from build123d import *

# Parameters (mm, degrees)
SKETCH1_W           = 14.15
SKETCH1_H           = 44.35
BOSS_EXTRUDE1_DEPTH = 1.19
SKETCH2_R           = 0.625
CUT_EXTRUDE1_DEPTH  = 24.306701826
SKETCH3_R           = 0.75
CUT_EXTRUDE2_DEPTH  = 24.306701826
SKETCH4_W           = 5
SKETCH4_H           = 4
BOSS_EXTRUDE2_DEPTH = 1.5
SKETCH4_3_W         = 1.75
SKETCH4_3_H         = 3.5
BOSS_EXTRUDE3_DEPTH = 1.65
SKETCH7_W           = 1.25
SKETCH7_H           = 2.5
BOSS_EXTRUDE6_DEPTH = 0.5


with BuildPart() as part:
    # Sketch1 → Boss-Extrude1 (new body)
    with BuildSketch(Plane(origin=(0, 0, 0), x_dir=(1, 0, 0), z_dir=(0, 1, 0))):
        Rectangle(SKETCH1_W, SKETCH1_H)
    extrude(amount=BOSS_EXTRUDE1_DEPTH)

    # Sketch2 → Cut-Extrude1 (cut, through all)
    with BuildSketch(Plane(origin=(0, 1.19, 0), x_dir=(1, 0, 0), z_dir=(0, 1, 0))):
        with Locations(Location((3.76, -20.635, 0), (0, 0, 270))):
            Circle(SKETCH2_R)
        with Locations(Location((1.253333333, -20.635, 0), (0, 0, 270))):
            Circle(SKETCH2_R)
        with Locations(Location((-1.253333333, -20.635, 0), (0, 0, 270))):
            Circle(SKETCH2_R)
        with Locations(Location((-3.76, -20.635, 0), (0, 0, 270))):
            Circle(SKETCH2_R)
    cut_extrude1 = extrude(amount=-CUT_EXTRUDE1_DEPTH, mode=Mode.SUBTRACT)

    # Mirror1: Cut-Extrude1 across plane
    add(cut_extrude1.mirror(Plane.XY), mode=Mode.SUBTRACT)

    # Sketch3 → Cut-Extrude2 (cut, through all)
    with BuildSketch(Plane(origin=(0, 1.19, 0), x_dir=(1, 0, 0), z_dir=(0, 1, 0))):
        with Locations(Location((2.56, -13.075, 0), (0, 0, 270))):
            Circle(SKETCH3_R)
        with Locations(Location((-2.56, -13.075, 0), (0, 0, 270))):
            Circle(SKETCH3_R)
    extrude(amount=-CUT_EXTRUDE2_DEPTH, mode=Mode.SUBTRACT)

    # Sketch4 → Boss-Extrude2 (add)
    with BuildSketch(Plane(origin=(0, 1.19, 0), x_dir=(1, 0, 0), z_dir=(0, 1, 0))):
        with Locations((2.075, 5.875)):
            Rectangle(SKETCH4_W, SKETCH4_H)
    extrude(amount=BOSS_EXTRUDE2_DEPTH)

    # Sketch4_3 → Boss-Extrude3 (add)
    with BuildSketch(Plane(origin=(0, 1.19, 0), x_dir=(1, 0, 0), z_dir=(0, 1, 0))):
        with Locations((-4.575, 5.875)):
            Rectangle(SKETCH4_3_W, SKETCH4_3_H)
    extrude(amount=BOSS_EXTRUDE3_DEPTH)

    # Sketch7 → Boss-Extrude6 (add)
    with BuildSketch(Plane(origin=(0, 1.19, 0), x_dir=(1, 0, 0), z_dir=(0, 1, 0))):
        with Locations((-4.575, -1.425)):
            Rectangle(SKETCH7_W, SKETCH7_H)
        with Locations((-1.525, -1.425)):
            Rectangle(SKETCH7_W, SKETCH7_H)
        with Locations((1.525, -1.425)):
            Rectangle(SKETCH7_W, SKETCH7_H)
        with Locations((4.575, -1.425)):
            Rectangle(SKETCH7_W, SKETCH7_H)
    boss_extrude6 = extrude(amount=BOSS_EXTRUDE6_DEPTH)

    # Mirror2: Boss-Extrude6 across plane
    add(boss_extrude6.mirror(Plane.XY.offset(-5.875)))


solid = part.part
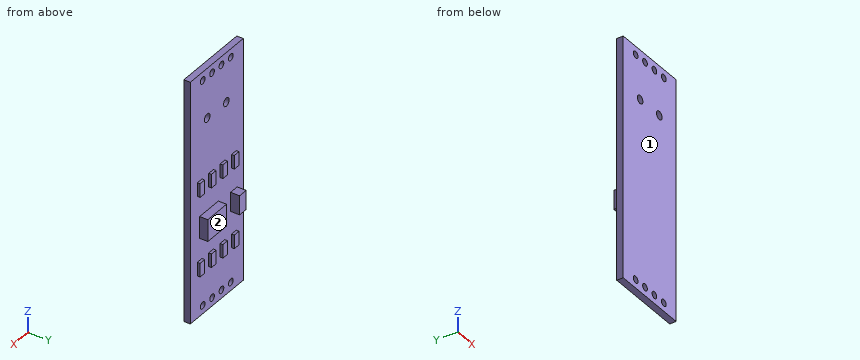
Can you work these out from the model? Positions are in its coordinate system, mm. Face numbers are marked on the shaded views. A direction names the side the tool comes from. Round coordinates to 2 decimals unless told otherwise and drop trailing zeros. Order: outer loops, then holes, each group sorted by start corner. A loop starts at its lowest first (then second) coordinate and runs counter-clockwise, first axis right, second up. Notation, with made-up numbers: (72.25, -36.75) - (108.25, -36.75) arc R6 ccw to (108.25, -31.75) - close; hole circle Ø11 at (-13.75, 73.5). An arc over 180 degrees is marked (long way). Answer in a Markdown table with one row per item.
(1) Suppose I cut it at B-B, the plane x = -2.56. Please give me the cut outline in (y, z) (3 decimals).
From the geometry:
| item | result |
|---|---|
| outline | (0, -22.175) - (1.19, -22.175) - (1.19, 12.325) - (0, 12.325) - close; (0, 13.825) - (1.19, 13.825) - (1.19, 22.175) - (0, 22.175) - close |
(2) For P1, Ø1, axis at x = 1.5, z = 1, coming from the +Y side; P2, Ø6, axis at x = -3.5, z = 16.5, coming from the +Y side, each with a flat end and sliding along its axis, tell me the tip position at first contact or that it passes through.
From the geometry:
| item | result |
|---|---|
| P1 | stops at y = 1.69 |
| P2 | stops at y = 1.19 |
(3) Which directions (+Z, -Z, +X, -X, +Y, -Y) give clear straight access to the entire face, cutting with the end or side of a thin tool? Please do the marked faces 1 and 2.
From the geometry:
| item | result |
|---|---|
| face 1 | +Z, -Z, +X, -X, -Y |
| face 2 | +Z, -Z, +X, +Y |
(4) Suppose I cut it at A-A, the plane y = 2.2. Please give me the cut outline in (x, z) (3 decimals).
From the geometry:
| item | result |
|---|---|
| outline | (-5.45, -7.625) - (-3.7, -7.625) - (-3.7, -4.125) - (-5.45, -4.125) - close; (-0.425, -7.875) - (4.575, -7.875) - (4.575, -3.875) - (-0.425, -3.875) - close |
(5) Suppose I cut it at C-C, the plane z = -11. Please give me the cut outline in (x, y) (3 decimals), plus the area to 3 significant figures.
From the geometry:
| item | result |
|---|---|
| outline | (-7.075, 0) - (7.075, 0) - (7.075, 1.19) - (-7.075, 1.19) - close |
| area | 16.8 mm2 |
(6) Suppose I cut it at D-D, the plane x = -6. Please give me the cut outline in (y, z) (3 decimals).
From the geometry:
| item | result |
|---|---|
| outline | (0, -22.175) - (1.19, -22.175) - (1.19, 22.175) - (0, 22.175) - close |
(7) Please list where these lines run through material, in increasing order: L1, parallel to Z at x = -2.5, y = 1.15 (3 decimals); L2, parallel to Y at x = -6.5, z = 5; L3, parallel to Z at x = -4, y = 1.8 (3 decimals). Write a range as from..to.
From the geometry:
| item | result |
|---|---|
| L1 | z = -22.175..12.327, 13.823..22.175 |
| L2 | y = 0..1.19 |
| L3 | z = -7.625..-4.125 |
